Work out the finished part from the listing and answer in its coordinate system (mm). Give positions to 0.01 mm unless a question says otherwise; leave off trailing zeros. Order: outer loops, then holes, each group sorted by start corner. A loop starts at its lowest first (then second) coordinate and runs counter-clockwise, first axis right, second up.
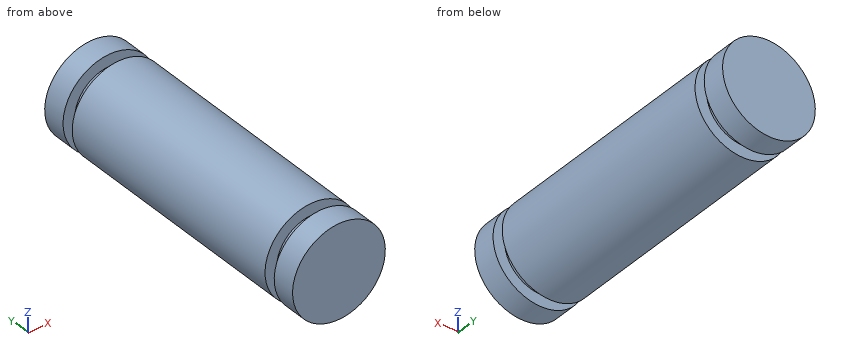
```python
from build123d import *

# Parameters (mm, degrees)
SKETCH1_R           = 4
BOSS_EXTRUDE1_DEPTH = 27
CUT_EXTRUDE1_START  = -3
SKETCH2_R           = 4
SKETCH2_R_2         = 3
CUT_EXTRUDE1_DEPTH  = 1
CUT_EXTRUDE2_START  = -25
SKETCH2_2_R         = 4
SKETCH2_2_R_2       = 3
CUT_EXTRUDE2_DEPTH  = 1


with BuildPart() as part:
    # Sketch1 → Boss-Extrude1 (new body)
    with BuildSketch(Plane(origin=(0, 0, 0), x_dir=(1, 0, 0), z_dir=(0, 1, 0))):
        with Locations(Location((0, 0, 0), (0, 0, 270))):
            Circle(SKETCH1_R)
    extrude(amount=BOSS_EXTRUDE1_DEPTH)

    # Sketch2 → Cut-Extrude1 (cut)
    with BuildSketch(Plane(origin=(0, 27, 0), x_dir=(1, 0, 0), z_dir=(0, 1, 0)).offset(CUT_EXTRUDE1_START)):
        with Locations(Location((0, 0, 0), (0, 0, 270))):
            Circle(SKETCH2_R)
        with Locations(Location((0, 0, 0), (0, 0, 270))):
            Circle(SKETCH2_R_2, mode=Mode.SUBTRACT)
    extrude(amount=CUT_EXTRUDE1_DEPTH, mode=Mode.SUBTRACT)

    # Sketch2_2 → Cut-Extrude2 (cut)
    with BuildSketch(Plane(origin=(0, 27, 0), x_dir=(1, 0, 0), z_dir=(0, 1, 0)).offset(CUT_EXTRUDE2_START)):
        with Locations(Location((0, 0, 0), (0, 0, 270))):
            Circle(SKETCH2_2_R)
        with Locations(Location((0, 0, 0), (0, 0, 270))):
            Circle(SKETCH2_2_R_2, mode=Mode.SUBTRACT)
    extrude(amount=CUT_EXTRUDE2_DEPTH, mode=Mode.SUBTRACT)


solid = part.part
```
1. The part is cut by section A-A (x = 0). Write down the section's boundary in (y, z), then the cut area to 3 significant figures.
Findings below:
outline: (0, -4) - (2, -4) - (2, -3) - (3, -3) - (3, -4) - (24, -4) - (24, -3) - (25, -3) - (25, -4) - (27, -4) - (27, 4) - (25, 4) - (25, 3) - (24, 3) - (24, 4) - (3, 4) - (3, 3) - (2, 3) - (2, 4) - (0, 4) - close
area: 212 mm2
2. The part is cut by section B-B (z = -3.25). Write down the section's boundary in (x, y).
Findings below:
outline: (-2.33, 0) - (2.33, 0) - (2.33, 2) - (-2.33, 2) - close; (-2.33, 3) - (2.33, 3) - (2.33, 24) - (-2.33, 24) - close; (-2.33, 25) - (2.33, 25) - (2.33, 27) - (-2.33, 27) - close
3. The part is cut by section C-C (z = 0). Write down the section's boundary in (x, y), then the cut area to 3 significant figures.
Findings below:
outline: (-4, 0) - (4, 0) - (4, 2) - (3, 2) - (3, 3) - (4, 3) - (4, 24) - (3, 24) - (3, 25) - (4, 25) - (4, 27) - (-4, 27) - (-4, 25) - (-3, 25) - (-3, 24) - (-4, 24) - (-4, 3) - (-3, 3) - (-3, 2) - (-4, 2) - close
area: 212 mm2
4. Straight lines are drawn through the part: probe 1 along Y at (x, z) = (3.5, -1.5); probe 2 along X at (y, z) = (4.75, 1.25); probe 3 along Z at (x, y) = (2.5, 5.25). For each, find the intervals that lie inside material, in ascending order.
Findings below:
probe 1: y = 0 to 2, 3 to 24, 25 to 27
probe 2: x = -3.8 to 3.8
probe 3: z = -3.12 to 3.12
5. Given P1, Ø1.5, axis at y = 5, z = -2.5, coming from the -X side; P2, Ø4, axis at x = -3, y = 14.5, coming from the +Z side, each flat-ended and moving along its own axis, determine where each tip first touches the part or whether it passes through.
Findings below:
P1: stops at x = -3.6
P2: stops at z = 3.87
6. The part is cut by section D-D (x = 3.5). Write down the section's boundary in (y, z).
Findings below:
outline: (0, -1.94) - (2, -1.94) - (2, 1.94) - (0, 1.94) - close; (3, -1.94) - (24, -1.94) - (24, 1.94) - (3, 1.94) - close; (25, -1.94) - (27, -1.94) - (27, 1.94) - (25, 1.94) - close
